Geometry check sheet. Reference: the model listing, model coordinates, mm. A direction names the side the tool comes from. Coordinates: 2 decimals unless noted, no trailing zeros. Write each loop counter-clockwise with the first axis right and the second up, starting at its lowest first coordinate (ties: lowest second). Pieces come first, ordered by that corner, then holes.
Autodesk Inventor part; units mm, degrees
ref_plane "YZ Plane" through (0, 0, 0) normal (1, 0, 0) x (0, 1, 0)
ref_plane "XZ Plane" through (0, 0, 0) normal (0, 1, 0) x (-1, 0, 0)
ref_plane "XY Plane" through (0, 0, 0) normal (0, 0, 1) x (1, 0, 0)
sketch "スケッチ1" plane through (0, 0, 0) normal (1, 0, 0) x (0, 1, 0)
  point P0 (0, 0)
sketch "スケッチ2" plane through (0, 0, 0) normal (1, 0, 0) x (0, 1, 0)
  line L0 (29.4185, 69.6387) -> (-30.5815, 69.6387)
  line L1 (-30.5815, 69.6387) -> (-30.5815, -70.3613)
  line L2 (-30.5815, -70.3613) -> (29.4185, -70.3613)
  line L3 (29.4185, -70.3613) -> (29.4185, 69.6387)
  point P0 (0, 0)
  dimension "d0" = 60
  dimension "d1" = 140
extrude "押し出し1" add sketch "スケッチ2" along normal blind 10
sketch "スケッチ3" plane through (0, 0, 0) normal (-1, 0, 0) x (0, 0, 1)
  circle A0 centre (-60.3613, 19.4185) radius 9
  line L0 (-70.3613, 29.4185) -> (69.6387, 29.4185)
  line L1 (-70.3613, -30.5815) -> (-70.3613, 29.4185)
  circle A1 centre (-60.3613, -20.5815) radius 9
  line L2 (69.6387, -30.5815) -> (-70.3613, -30.5815)
  circle A2 centre (59.6387, -20.5815) radius 9
  line L3 (69.6387, 29.4185) -> (69.6387, -30.5815)
  circle A3 centre (59.6387, 19.4185) radius 9
  circle A4 centre (-60.3613, 19.4185) radius 8
  circle A5 centre (-60.3613, -20.5815) radius 8
  circle A6 centre (59.6387, 19.4185) radius 8
  circle A7 centre (59.6387, -20.5815) radius 8
  point P0 (0, 0)
  dimension "d4" = 18
  dimension "d5" = 10
  dimension "d6" = 10
  dimension "d7" = 18
  dimension "d8" = 10
  dimension "d9" = 18
  dimension "d10" = 10
  dimension "d11" = 18
  dimension "d12" = 16
  dimension "d13" = 16
  dimension "d14" = 16
  dimension "d15" = 16
extrude "押し出し2" add sketch "スケッチ3" along normal blind 10 contours A0 | A1 | A2 | A3
sketch "スケッチ4" plane through (0, 0, 0) normal (-1, 0, 0) x (0, 0, 1)
  point P0 (0, 0)
sketch "スケッチ5" plane through (0, 0, 0) normal (-1, 0, 0) x (0, 0, 1)
  circle A0 centre (-60.3613, 19.4185) radius 3
  line L0 (-70.3613, 29.4185) -> (69.6387, 29.4185)
  line L1 (-70.3613, -30.5815) -> (-70.3613, 29.4185)
  circle A1 centre (-60.3613, -20.5815) radius 3
  line L2 (69.6387, -30.5815) -> (-70.3613, -30.5815)
  circle A2 centre (59.6387, 19.4185) radius 3
  line L3 (69.6387, 29.4185) -> (69.6387, -30.5815)
  point P0 (0, 0)
  dimension "d18" = 6
  dimension "d19" = 10
  dimension "d20" = 10
  dimension "d21" = 6
  dimension "d22" = 10
  dimension "d23" = 6
  dimension "d24" = 10
sketch "スケッチ6" plane through (0, 0, 0) normal (-1, 0, 0) x (0, 0, 1)
  circle A0 centre (-60.3613, 19.4185) radius 3
  circle A1 centre (59.6387, 19.4185) radius 3
  circle A2 centre (59.6387, -20.5815) radius 3
  line L0 (69.6387, 29.4185) -> (69.6387, -30.5815)
  line L1 (69.6387, -30.5815) -> (-70.3613, -30.5815)
  point P0 (0, 0)
  dimension "d25" = 6
  dimension "d26" = 6
  dimension "d27" = 6
  dimension "d28" = 10
  dimension "d29" = 10
extrude "押し出し3" add sketch "スケッチ6" along normal blind 28
extrude "押し出し4" add sketch "スケッチ5" along normal blind 28 contours A1
sketch "スケッチ7" plane through (10, 0, 0) normal (1, 0, 0) x (0, 0, -1)
  point P0 (0, 0)
sketch "スケッチ8" plane through (10, 0, 0) normal (1, 0, 0) x (0, 0, -1)
  circle A0 centre (0, 0) radius 1
  dimension "d35" = 2
sketch "スケッチ9" plane through (10, 0, 0) normal (1, 0, 0) x (0, 0, -1)
  circle A0 centre (0, 0) radius 3
  dimension "d36" = 6
hole "穴1" at (10, 0, 0) direction (-1, 0, 0) diameter 6 depth 10
equation "\"BendRadius\" = Thickness"
equation "\"BendReliefWidth\" = Thickness"
equation "\"BendReliefDepth\" = 0.5 * Thickness"
equation "\"CornerReliefSize\" = 4 * Thickness"
equation "\"MinimumRemnant\" = 2 * Thickness"
equation "\"TransitionRadius\" = BendRadius"
equation "\"JacobiRadiusSize\" = BendRadius"
equation "\"GapSize\" = Thickness"
1. Sectioned sample at A-A, the plane y = 0. Record the boundary of the cut face in (x, z).
Computed values:
outline: (0, -70.36) - (10, -70.36) - (10, -3) - (0, -3) - close; (0, 3) - (10, 3) - (10, 69.64) - (0, 69.64) - close
2. Sectioned sample at C-C, the plane x = -8. Give the number of separate pieces and of enclosed holes in the cut face, and give its area (3 significant figures).
Computed values:
separate pieces: 8
enclosed holes: 4
area: 327 mm2
3. Access from +Z, -Z, +X, -X, +Y, -Y to the whole of each face (thin tool, end or side, straight path). Record for faces 4 (the cylindrical face through (-4.93, -20.977, -69.353)), 5 (the flat face through (5, -1, -70.361)).
Computed values:
face 4: -X
face 5: -Z, +X, -X, +Y, -Y
4. Thickness scan on line 1 along Z through (x, y) = (-3.5, 24.5); line 2 along Z through (x, y) = (-3, -23); line 3 along X through (y, z) = (19.5, 25.5). Record the ranges inside material, lowest first.
Computed values:
line 1: z = -67.79 to -66.54, -54.18 to -52.93, 52.21 to 53.46, 65.82 to 67.07
line 2: z = -69.03 to -67.99, -62.14 to -58.59, -52.74 to -51.69, 50.97 to 52.01, 57.86 to 61.41, 67.26 to 68.31
line 3: x = 0 to 10
5. Draft check along Y on faces 1 (the flat face through (-28, 19, -60)), 2 (the flat face through (5, 29.418, -1)), 3 (the flat face through (-10, 13, -66)). Enter one of: released by +Y, released by -Y, zero draft, split by the parting line, or undercut.
Computed values:
face 1: zero draft
face 2: released by +Y
face 3: undercut
6. Gauge pin test, flat ends, axial feed: pin 1 Ø1.5 at (y, z) = (-22.5, 42) entering from -X; pin 2 Ø5 at (x, y) = (-21.5, -18) entering from +Z. Record the tip position at first contact, or that the pin passes through.
Computed values:
pin 1: stops at x = 0
pin 2: stops at z = 62.64
7. Sectioned sample at D-D, the plane y = -26. Record the boundary of the cut face in (x, z).
Computed values:
outline: (-10, -67.55) - (0, -67.55) - (0, -70.36) - (10, -70.36) - (10, 69.64) - (0, 69.64) - (0, 66.82) - (-10, 66.82) - (-10, 65.52) - (0, 65.52) - (0, 53.75) - (-10, 53.75) - (-10, 52.45) - (0, 52.45) - (0, -53.18) - (-10, -53.18) - (-10, -54.48) - (0, -54.48) - (0, -66.25) - (-10, -66.25) - close
8. Sectioned sample at B-B, the plane z = 0. Record the boundary of the cut face in (x, y).
Computed values:
outline: (0, -30.58) - (10, -30.58) - (10, -3) - (0, -3) - close; (0, 3) - (10, 3) - (10, 29.42) - (0, 29.42) - close
